from build123d import *

# Parameters (mm, degrees)
SKETCH1_R      = 4.7625
EXTRUDE1_DEPTH = 1.5


with BuildPart() as part:
    # Sketch1 → Extrude1 (new body)
    with BuildSketch(Plane.XY.offset(165.1)):
        with BuildLine():
            Line((-418.175, 962.43), (-554.955743448, 962.43))
            ThreePointArc((-554.955743448, 962.43), (-529.269854117, 938.688748088), (-519.775, 905.024825288))
            Line((-519.775, 905.024825288), (-519.775, 813.93))
            ThreePointArc((-519.775, 813.93), (-512.335512242, 795.969487758), (-494.375, 788.53))
            Line((-494.375, 788.53), (-418.175, 788.53))
            Line((-418.175, 788.53), (-418.175, 962.43))
        make_face()
        with Locations((-444.2625, 801.23)):
            Circle(SKETCH1_R, mode=Mode.SUBTRACT)
        with Locations((-495.0625, 801.23)):
            Circle(SKETCH1_R, mode=Mode.SUBTRACT)
    extrude(amount=EXTRUDE1_DEPTH)


solid = part.part
CAD build for the part. Positions are in the model's coordinates, mm. Give positions to 0.01 mm unless a question says otherwise; leave off trailing zeros. Loops run counter-clockwise (first coordinate to the right, second up) from the corner with the lowest first, then second, coordinate; pieces in that order, holes last. Notation, with made-up numbers: M 7,0 L 21,0 A31 cw 21,28 Z; hole C 19.25,57 d5. An arc over 180 degrees is marked long. Answer in a Markdown table with one row per item. Add a question column.
Item 1: Probe probe 1 along X at (y, z) = (801.23, 165.9) (3 decimals); probe 2 along X at (y, z) = (877, 166.5) (3 decimals); probe 3 along Y at (x, z) = (-501, 165.35). List the from-to ranges inside material, lowest first.
Item 2: Band-saw the part on A-A on z = 166.25. Give the number of separate pieces and of enclosed holes in the cut face, then the cut area to 3 significant figures.
Item 3: Band-saw the part on B-B on y = 801.23. Give the cut face in (x, z) (3 decimals), then the cut area to 3 significant figures.
Item 4: Mould opens along Y. For faces 1 (the face through (-492.865, 797.005, 165.84)), 2 (the face through (-529.53, 939.11, 165.84)), 3 (the face through (-472, 877, 166.6)) say: +Y half, -Y half, draft (parallel to the pull), parting line (faces both ways), or undercut.
Item 5: Band-saw the part on C-C on y = 868. Give the cut face in (x, z) (3 decimals), then the cut area to 3 significant figures.
Item 6: Band-saw the part on D-D on y = 931.5. Give the cut face in (x, z) (3 decimals), then the cut area to 3 significant figures.
Reply:
| question | item | result |
|---|---|---|
| 1 | probe 1 | x = -516.372 to -499.825, -490.3 to -449.025, -439.5 to -418.175 |
| 1 | probe 2 | x = -519.775 to -418.175 |
| 1 | probe 3 | y = 789.41 to 962.43 |
| 2 | separate pieces | 1 |
| 2 | enclosed holes | 2 |
| 2 | area | 18,000 mm^2 |
| 3 | outline | M -516.372,165.1 L -499.825,165.1 L -499.825,166.6 L -516.372,166.6 Z; M -490.3,165.1 L -449.025,165.1 L -449.025,166.6 L -490.3,166.6 Z; M -439.5,165.1 L -418.175,165.1 L -418.175,166.6 L -439.5,166.6 Z |
| 3 | area | 119 mm^2 |
| 4 | face 1 | undercut |
| 4 | face 2 | -Y half |
| 4 | face 3 | draft |
| 5 | outline | M -519.775,165.1 L -418.175,165.1 L -418.175,166.6 L -519.775,166.6 Z |
| 5 | area | 152 mm^2 |
| 6 | outline | M -525.466,165.1 L -418.175,165.1 L -418.175,166.6 L -525.466,166.6 Z |
| 6 | area | 161 mm^2 |
